The figure shows three views and two pictorial views of one solid part (mm, origin at its lowest corner). Answer the questions. A direction names the side the tool comes from. Coordinates: 2 decimals unless noted, no trailing zeros. Order: outer loops, then holes, each group sorted by start corner. A loop starts at its lowest first (then second) coordinate and runs counter-clockwise, first axis right, second up. Notation, with made-up numbers: (-0.75, 52.25) -> (6.25, 52.25) arc R15 cw to (6.25, 64.25) -> close; hole circle Ø6 at (15.25, 40.5). An arc over 180 degrees is marked (long way). Use one line per item in the form item = value.
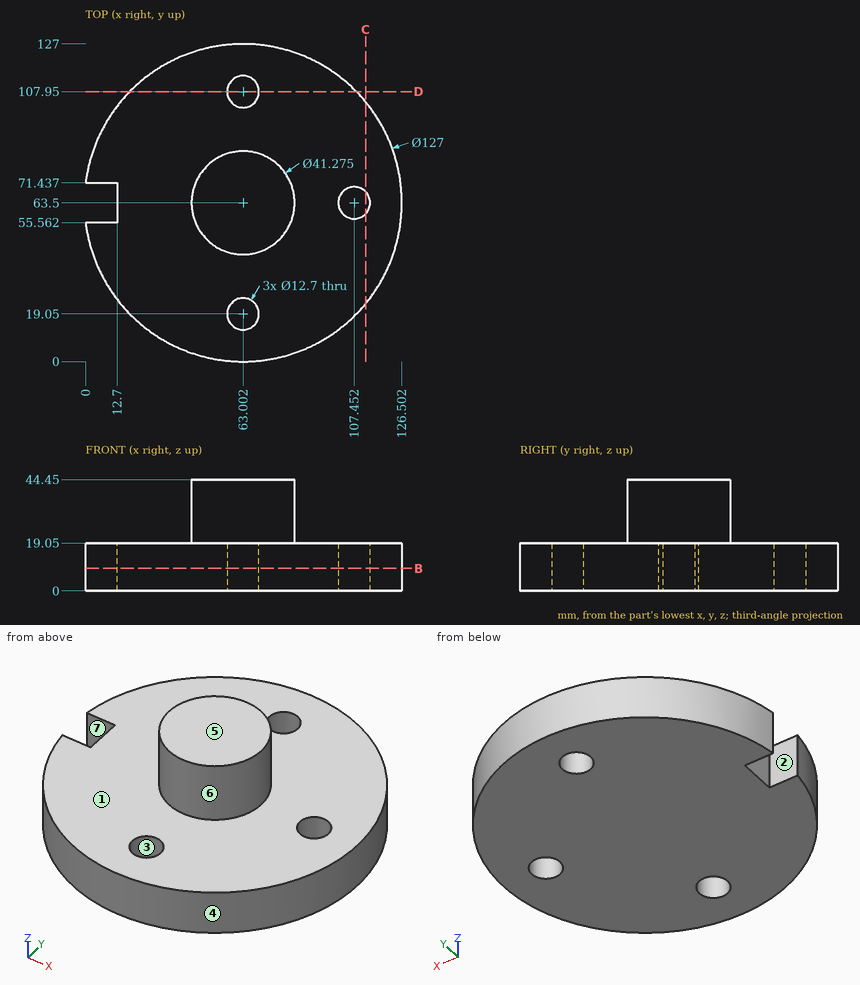
(1) Section C-C on x = 112 is taken. Write down the section's boundary in (y, z), plus the area to 3 significant figures.
Data:
outline = (23.11, 0) -> (59.07, 0) -> (59.07, 19.05) -> (23.11, 19.05) -> close; (67.93, 0) -> (103.89, 0) -> (103.89, 19.05) -> (67.93, 19.05) -> close
area = 1,370 mm²
(2) Which of the six approach directions +Z, -Z, +X, -X, +Y, -Y give full straight-line access (tool end or side, diameter ignored) to the marked faces 5, 6 and 7?
Data:
face_5 = +Z, +X, -X, +Y, -Y
face_6 = +Z
face_7 = +Z, -Z, -X
(3) Section D-D on y = 107.95 is taken. Write down the section's boundary in (x, z), plus the area to 3 significant figures.
Data:
outline = (17.65, 0) -> (56.65, 0) -> (56.65, 19.05) -> (17.65, 19.05) -> close; (69.35, 0) -> (108.35, 0) -> (108.35, 19.05) -> (69.35, 19.05) -> close
area = 1,490 mm²
(4) Section B-B on z = 9 is taken. Write down the section's boundary in (x, y), plus the area to 3 significant figures.
Data:
outline = (0, 55.56) arc R63.5 ccw (long way) to (0, 71.44) -> (12.7, 71.44) -> (12.7, 55.56) -> close; hole circle Ø12.7 at (63, 19.05); hole circle Ø12.7 at (63, 107.95); hole circle Ø12.7 at (107.45, 63.5)
area = 12,100 mm²
(5) Each of these flat-tipped pins is pushed along its axis until it touches: P1, Ø6, axis at x = 79.5, z = 22.5, coming from the -Y side; P2, Ø4, axis at y = 79, z = 27, coming from the +X side; P3, Ø10, axis at x = 91.5, z = 15.5, coming from the +Y side; P4, Ø3, axis at x = 92.5, z = 22, coming from the +Y side. Where does it stop, or does it pass through?
Data:
P1 = 47.89
P2 = 78.61
P3 = 122.49
P4 = through
(6) Straight lines are drawn through the part: line 1 along X through (y, z) = (63.5, 4.5); line 2 along Z through (x, y) = (35.5, 51); line 3 along X through (y, z) = (107, 5) (1 decimal). For each, find the intervals that lie inside material, in ascending order.
Data:
line_1 = 12.7 to 101.1, 113.8 to 126.5
line_2 = 0 to 19.05
line_3 = 16.7 to 56.7, 69.3 to 109.3
(7) The mould has two halves that part along Y. Classify the marked faces 1, 2, 3 and 4: released by +Y, released by -Y, zero draft, split by the parting line, or undercut.
Data:
face_1 = zero draft
face_2 = undercut
face_3 = undercut
face_4 = split by the parting line
